```python
from build123d import *

# Parameters (mm, degrees)
BOSS_EXTRUDE1_DEPTH = 5
SKETCH4_R           = 1.5
CUT_EXTRUDE1_DEPTH  = 91.518644488
SKETCH6_R           = 5.35
BOSS_EXTRUDE2_DEPTH = 1.5
CUT_EXTRUDE2_REACH  = 92.614
SKETCH7_R           = 1.5
CUT_EXTRUDE3_START  = -5
CUT_EXTRUDE3_DEPTH  = 5


# Read off the part's stored shape, not the designer's step: Cut-Extrude3
with BuildPart() as part:
    # Sketch3 → Boss-Extrude1 (new body)
    with BuildSketch(Plane(origin=(0, 0, 0), x_dir=(1, 0, 0), z_dir=(0, 1, 0))):
        with BuildLine():
            Line((-75, 14.25), (75, 14.25))
            ThreePointArc((75, 14.25), (89.25, 0), (75, -14.25))
            Line((75, -14.25), (-75, -14.25))
            ThreePointArc((-75, -14.25), (-89.25, 0), (-75, 14.25))
        make_face()
    extrude(amount=BOSS_EXTRUDE1_DEPTH)

    # Sketch4 → Cut-Extrude1 (cut, through all)
    with BuildSketch(Plane(origin=(0, 5, 0), x_dir=(1, 0, 0), z_dir=(0, 1, 0))):
        with Locations(Location((25, 0, 0), (0, 0, 270))):
            Circle(SKETCH4_R)
        with Locations(Location((75, 0, 0), (0, 0, 270))):
            Circle(SKETCH4_R)
    extrude(amount=-CUT_EXTRUDE1_DEPTH, mode=Mode.SUBTRACT)

    # Sketch6 → Boss-Extrude2 (add)
    with BuildSketch(Plane.XZ):
        with Locations(Location((75, 0, 0), (0, 0, 90))):
            Circle(SKETCH6_R)
    extrude(amount=BOSS_EXTRUDE2_DEPTH)

    # Sketch7 → Cut-Extrude2 (cut, up to next)
    with BuildSketch(Plane.XZ.offset(1.5), mode=Mode.PRIVATE) as cut_extrude2_sk1:
        with Locations(Location((75, 0, 0), (0, 0, 90))):
            Circle(SKETCH7_R)
    cut_extrude2_tool1 = extrude(cut_extrude2_sk1.sketch, amount=-CUT_EXTRUDE2_REACH, mode=Mode.PRIVATE) & part.part
    add(cut_extrude2_tool1.solids().sort_by_distance((75, -1.5, 0))[0], mode=Mode.SUBTRACT)

    # Cut-Extrude3 outline → Cut-Extrude3 (cut)
    with BuildSketch(Plane.XZ.offset(CUT_EXTRUDE3_START)):
        with BuildLine():
            add(Edge.make_bspline(
                [(78.847956131, 3.716952194), (76.072393782, 6.590339205), (61.349969699, 12.082853178), (43.710632326, 14.25), (39.933768596, 14.25)],
                knots=[0, 0, 0, 0, 0.424659956, 1, 1, 1, 1], degree=3))
            ThreePointArc((78.847956131, 3.716952194), (79.924844883, -2.090072458), (75, -5.35))
            add(Edge.make_bspline(
                [(-34.598022438, -14.25), (-16.711424767, -14.25), (16.96977211, -7.115763951), (68.517114085, -5.35), (75, -5.35)],
                knots=[0, 0, 0, 0, 0.557363476, 1, 1, 1, 1], degree=3))
            Line((-34.598022438, -14.25), (75, -14.25))
            ThreePointArc((75, -14.25), (89.25, 0), (75, 14.25))
            Line((75, 14.25), (39.933768596, 14.25))
        make_face()
    extrude(amount=CUT_EXTRUDE3_DEPTH, mode=Mode.SUBTRACT)


solid = part.part
```
CAD build for the part. Positions are in the model's coordinates, mm. Coordinates: 2 decimals unless noted, no trailing zeros. Write each loop counter-clockwise with the first axis right and the second up, starting at its lowest first coordinate (ties: lowest second). Pieces come first, ordered by that corner, then holes.
(1) Cut at C-C, the plane x = -61. List the corners of the cut face in (y, z), and give its area (4 significant figures).
(2) Cut at B-B, the plane y = 2.75. Count the separate pieces of the cut face and the enclosed holes in it, and give its area (3 significant figures).
(3) Two-plate mould, pull along Z, no slides. Class faces 1 (the face through (76.1, -1.5, -1.3)), 2 (the face through (26.487, 2.535, -0.195)), 3 (the face through (-55, 2, -14.25)), 4 (the face through (73.735, 1.704, 0.806)): +Z half, -Z half, draft (parallel to the pull), parting line (faces both ways), or undercut.
(4) Cut at A-A, the plane z = 0. List the corners of the cut face in (x, y).
(5) Flat gauge pins, fed straight in: pin 1 (6 mm diameter, centred on x = -46, z = 6.5, fed in from -Y); pin 2 (1 mm diameter, centred on x = 10.5, y = 0.5, fed in from -Z). Where does each tip first touch, or does it go through?
(6) Drill centre lines: probe 1 along X at (y, z) = (1.5, 0); probe 2 along Y at (x, z) = (-49, 10.5); probe 3 along Z at (x, y) = (75, 2.5). Where is each one in solid material? Low to high.
Geometry says:
1. outline: (0, -14.25) - (5, -14.25) - (5, 14.25) - (0, 14.25) - close
1. area: 142.5 mm2
2. separate pieces: 1
2. enclosed holes: 2
2. area: 3,980 mm2
3. face 1: draft
3. face 2: undercut
3. face 3: -Z half
3. face 4: undercut
4. outline: (-89.25, 0) - (23.5, 0) - (23.5, 5) - (-89.25, 5) - close; (26.5, 0) - (69.65, 0) - (69.65, -1.5) - (73.5, -1.5) - (73.5, 5) - (26.5, 5) - close; (76.5, -1.5) - (80.35, -1.5) - (80.35, 5) - (76.5, 5) - close
5. pin 1: stops at y = 0
5. pin 2: stops at z = -9.81
6. probe 1: x = -89.25 to 23.5, 26.5 to 73.5, 76.5 to 80.35
6. probe 2: y = 0 to 5
6. probe 3: z = -5.35 to -1.5, 1.5 to 6.42
